from build123d import *

# Parameters (mm, degrees)
SKETCH1_R           = 28.575
BOSS_EXTRUDE1_DEPTH = 5.08
SKETCH2_W           = 25.4
SKETCH2_H           = 5.08
BOSS_EXTRUDE2_DEPTH = 63.5
SKETCH3_R           = 24.257
CUT_EXTRUDE1_DEPTH  = 50.8
SKETCH4_W           = 5.08
SKETCH4_H           = 19.05
CUT_EXTRUDE2_DEPTH  = 50.8
SKETCH6_W           = 5.08
SKETCH6_H           = 37.902331649
BOSS_EXTRUDE4_DEPTH = 19.05
SKETCH7_W           = 5.08
SKETCH7_H           = 19.05
CUT_EXTRUDE3_DEPTH  = 25.4
FILLET1_R           = 12.7
SKETCH8_W           = 5.08
SKETCH8_H           = 6.35
BOSS_EXTRUDE5_DEPTH = 23.495


with BuildPart() as part:
    # Sketch1 → Boss-Extrude1 (new body)
    with BuildSketch(Plane.XY):
        Circle(SKETCH1_R)
    extrude(amount=BOSS_EXTRUDE1_DEPTH)

    # Sketch2 → Boss-Extrude2 (add)
    with BuildSketch(Plane(origin=(0, 0, 0), x_dir=(1, 0, 0), z_dir=(0, 1, 0))):
        with Locations((0, -2.54)):
            Rectangle(SKETCH2_W, SKETCH2_H)
    extrude(amount=BOSS_EXTRUDE2_DEPTH)

    # Sketch3 → Cut-Extrude1 (cut)
    with BuildSketch(Plane(origin=(0, 0, 0), x_dir=(-1, 0, 0), z_dir=(0, 0, -1))):
        Circle(SKETCH3_R)
    extrude(amount=-CUT_EXTRUDE1_DEPTH, mode=Mode.SUBTRACT)

    # Sketch4 → Cut-Extrude2 (cut)
    with BuildSketch(Plane(origin=(0, 0, 0), x_dir=(-1, 0, 0), z_dir=(0, 0, -1))):
        with Locations((0, 41.275)):
            Rectangle(SKETCH4_W, SKETCH4_H)
    extrude(amount=-CUT_EXTRUDE2_DEPTH, mode=Mode.SUBTRACT)

    # Sketch6 → Boss-Extrude4 (add)
    with BuildSketch(Plane(origin=(12.7, 0, 0), x_dir=(0, 0, -1), z_dir=(1, 0, 0))):
        with Locations((-2.54, 44.548834176)):
            Rectangle(SKETCH6_W, SKETCH6_H)
    extrude(amount=BOSS_EXTRUDE4_DEPTH)

    # Sketch7 → Cut-Extrude3 (cut)
    with BuildSketch(Plane.XY.offset(5.08)):
        with Locations((10.16, 41.275)):
            Rectangle(SKETCH7_W, SKETCH7_H)
    extrude(amount=-CUT_EXTRUDE3_DEPTH, mode=Mode.SUBTRACT)

    # Fillet1
    fillet1_edges = [part.edges().sort_by_distance(p)[0] for p in [
        (-12.7, 63.5, 2.54),
        (31.75, 63.5, 2.54),
        (31.75, 25.597668351, 2.54),
    ]]
    fillet(fillet1_edges, radius=FILLET1_R)

    # Sketch8 → Boss-Extrude5 (add)
    with BuildSketch(Plane(origin=(31.75, 0, 0), x_dir=(0, 0, -1), z_dir=(1, 0, 0))):
        with Locations((-2.54, 44.2518817)):
            Rectangle(SKETCH8_W, SKETCH8_H)
    extrude(amount=BOSS_EXTRUDE5_DEPTH)


solid = part.part
Verification items for the finished model (mm, model axes). A direction names the side the tool comes from. Give positions to 0.01 mm unless a question says otherwise; leave off trailing zeros. Write each loop counter-clockwise with the first axis right and the second up, starting at its lowest first coordinate (ties: lowest second). Pieces come first, ordered by that corner, then holes. Notation, with made-up numbers: M -26.5,25.5 L 29.5,25.5 A19 cw 29.5,38.5 Z; hole C 55,-23 d6. An arc over 180 degrees is marked long. Write item = value, one per line.
(1) Material ranges on line 1 (Y direction, x = 0, z = 3.75) (3 decimals); line 2 (Y direction, x = 42.5, z = 0.8); line 3 (Y direction, x = -6, z = 4), recorded low to high.
Found:
line_1 = -28.575 to -24.257, 24.257 to 31.75, 50.8 to 63.5
line_2 = 41.08 to 47.43
line_3 = -27.94 to -23.5, 23.5 to 61.99
(2) Go/stop test with flat-tipped pins: pin 1 Ø3 at (x, z) = (39, 1.5) entering from +Y; pin 2 Ø1 at (x, y) = (22.5, 0.5) entering from +Z; pin 3 Ø2.5 at (x, z) = (16, 3) entering from -Y; pin 4 Ø3 at (x, z) = (-5, 3) entering from +Y. Record where each tip stops, or that it passes through.
Found:
pin_1 = 47.43
pin_2 = through
pin_3 = -24.47
pin_4 = 63.01
(3) Access from +Z, -Z, +X, -X, +Y, -Y to the whole of each face (thin tool, end or side, straight path). Record for faces 1 (the face through (31.75, 40, 3)), 2 (the face through (0, 31.75, 3)), 3 (the face through (27.93, 29.22, 2.5)), 4 (the face through (43, 47.427, 3)), 5 (the face through (-9.08, 59.68, 2.5)).
Found:
face_1 = +Z, -Z, +X, -Y
face_2 = +Z, -Z
face_3 = +Z, -Z, +X
face_4 = +Z, -Z, +X, +Y
face_5 = +Z, -Z, -X, +Y
(4) Sectioned sample at B-B (z = 0.8). Record the cut outline in (x, y) (3 decimals), then the cut area to 3 significant figures.
Found:
outline = M -12.7,25.598 A28.575 ccw long 12.7,25.598 L 19.05,25.598 A12.7 ccw 31.75,38.298 L 31.75,41.077 L 55.245,41.077 L 55.245,47.427 L 31.75,47.427 L 31.75,50.8 A12.7 ccw 19.05,63.5 L 0,63.5 A12.7 ccw -12.7,50.8 Z; hole C 0,0 d48.514; hole M -2.54,31.75 L 2.54,31.75 L 2.54,50.8 L -2.54,50.8 Z; hole M 7.62,31.75 L 12.7,31.75 L 12.7,50.8 L 7.62,50.8 Z
area = 2,200 mm2
(5) Draft check along X on faces 6 (the face through (43, 41.077, 3)), 7 (the face through (28.13, 59.68, 2.5)), 8 (the face through (10, 50.8, 3)), 9 (the face through (-12.7, 38, 3)). Enter one of: released by +X, released by -X, zero draft, split by the parting line, or undercut.
Found:
face_6 = zero draft
face_7 = released by +X
face_8 = undercut
face_9 = released by -X
(6) Sectioned sample at A-A (y = 0). Record the cut outline in (x, z) (3 decimals).
Found:
outline = M -28.575,0 L -24.257,0 L -24.257,5.08 L -28.575,5.08 Z; M 24.257,0 L 28.575,0 L 28.575,5.08 L 24.257,5.08 Z
(7) Sectioned sample at C-C (x = -20.5). Record the cut outline in (y, z).
Found:
outline = M -19.91,0 L -12.97,0 L -12.97,5.08 L -19.91,5.08 Z; M 12.97,0 L 19.91,0 L 19.91,5.08 L 12.97,5.08 Z
(8) Sectioned sample at D-D (y = 39.5). Record the cut outline in (x, z).
Found:
outline = M -12.7,0 L -2.54,0 L -2.54,5.08 L -12.7,5.08 Z; M 2.54,0 L 7.62,0 L 7.62,5.08 L 2.54,5.08 Z; M 12.7,0 L 31.75,0 L 31.75,5.08 L 12.7,5.08 Z
